```python
from build123d import *

# Parameters (mm, degrees)
F1_DEPTH = 273.05
F2_DEPTH = 6.35
F4_DEPTH = 25.4
F5_W     = 20.32
F5_H     = 203.2
F6_DEPTH = 21.082
F7_R     = 3.175


with BuildPart() as f1:
    # F0 (on Front) → F1 (new body)
    with BuildSketch(Plane.XZ):
        with BuildLine():
            Line((15.875, -3.175), (15.55426, -3.175))
            ThreePointArc((15.55426, -3.175), (10.040232, -12.296722), (0, -15.875))
            Line((0, -15.875), (0, -26.67))
            ThreePointArc((0, -26.67), (8.358623, -25.326317), (15.875, -21.430662))
            Line((15.875, -21.430662), (15.875, -3.175))
        make_face()
        with BuildLine():
            ThreePointArc((0, -15.875), (-10.040232, -12.296722), (-15.55426, -3.175))
            Line((-15.55426, -3.175), (-15.875, -3.175))
            Line((-15.875, -3.175), (-15.875, -21.430662))
            ThreePointArc((-15.875, -21.430662), (-8.358623, -25.326317), (0, -26.67))
            Line((0, -26.67), (0, -15.875))
        make_face()
        with BuildLine():
            ThreePointArc((15.875, -21.430662), (8.358623, -25.326317), (0, -26.67))
            Line((0, -26.67), (0, -27.432))
            ThreePointArc((0, -27.432), (4.143033, -27.930592), (8.049481, -29.397895))
            ThreePointArc((8.049481, -29.397895), (12.080918, -27.983599), (15.875, -26.019508))
            Line((15.875, -26.019508), (15.875, -21.430662))
        make_face()
        with BuildLine():
            ThreePointArc((-8.049481, -29.397895), (-12.080918, -27.983599), (-15.875, -26.019508))
            Line((-15.875, -26.019508), (-15.875, -34.925))
            Line((-15.875, -34.925), (-14.336944, -34.925))
            ThreePointArc((-14.336944, -34.925), (-11.529321, -31.779102), (-8.049481, -29.397895))
        make_face()
        with BuildLine():
            Line((0, -27.432), (0, -26.67))
            ThreePointArc((0, -26.67), (-8.358623, -25.326317), (-15.875, -21.430662))
            Line((-15.875, -21.430662), (-15.875, -26.019508))
            ThreePointArc((-15.875, -26.019508), (-12.080918, -27.983599), (-8.049481, -29.397895))
            ThreePointArc((-8.049481, -29.397895), (-4.143033, -27.930592), (0, -27.432))
        make_face()
        with BuildLine():
            Line((15.875, -34.925), (15.875, -26.019508))
            ThreePointArc((15.875, -26.019508), (12.080918, -27.983599), (8.049481, -29.397895))
            ThreePointArc((8.049481, -29.397895), (11.529321, -31.779102), (14.336944, -34.925))
            Line((14.336944, -34.925), (15.875, -34.925))
        make_face()
        with BuildLine():
            ThreePointArc((0, -12.7), (-7.77713, -10.040232), (-12.296722, -3.175))
            Line((-12.296722, -3.175), (-15.55426, -3.175))
            ThreePointArc((-15.55426, -3.175), (-10.040232, -12.296722), (0, -15.875))
            Line((0, -15.875), (0, -12.7))
        make_face()
        with BuildLine():
            Line((15.55426, -3.175), (12.296722, -3.175))
            ThreePointArc((12.296722, -3.175), (7.77713, -10.040232), (0, -12.7))
            Line((0, -12.7), (0, -15.875))
            ThreePointArc((0, -15.875), (10.040232, -12.296722), (15.55426, -3.175))
        make_face()
    extrude(amount=F1_DEPTH)

    # F0 (on Front) → F2 (join)
    with BuildSketch(Plane.XZ):
        with BuildLine():
            ThreePointArc((0, -12.7), (-7.77713, -10.040232), (-12.296722, -3.175))
            Line((-12.296722, -3.175), (-15.55426, -3.175))
            ThreePointArc((-15.55426, -3.175), (-10.040232, -12.296722), (0, -15.875))
            Line((0, -15.875), (0, -12.7))
        make_face()
        with BuildLine():
            Line((15.55426, -3.175), (12.296722, -3.175))
            ThreePointArc((12.296722, -3.175), (7.77713, -10.040232), (0, -12.7))
            Line((0, -12.7), (0, -15.875))
            ThreePointArc((0, -15.875), (10.040232, -12.296722), (15.55426, -3.175))
        make_face()
    extrude(amount=-F2_DEPTH)

    # F3 (on Right) → F4 (cut, symmetric)
    with BuildSketch(Plane.YZ):
        with BuildLine():
            Line((-285.688049, -3.085141), (-285.688049, -18.728113))
            Line((-285.688049, -18.728113), (-107.888049, -18.728113))
            add(Edge.make_bspline(
                [(-18.988049, -3.085141), (-51.164284, -4.672805), (-75.452253, -18.588752), (-107.888049, -18.728113)],
                knots=[0, 0, 0, 0, 90.265789, 90.265789, 90.265789, 90.265789], degree=3))
            Line((-18.988049, -3.085141), (-285.688049, -3.085141))
        make_face()
    extrude(amount=F4_DEPTH, both=True, mode=Mode.SUBTRACT)

    # F5 (on Top) → F6 (cut)
    with BuildSketch(Plane.XY):
        with Locations((0, -127)):
            Rectangle(F5_W, F5_H)
    extrude(amount=-F6_DEPTH, mode=Mode.SUBTRACT)

    # F7
    f7_edges = [f1.edges().sort_by_distance(p)[0] for p in [
        (-10.16, -25.4, -14.351),
        (10.16, -25.4, -14.351),
        (-10.16, -228.6, -19.905056),
        (10.16, -228.6, -19.905056),
    ]]
    fillet(f7_edges, radius=F7_R)


solid = f1.part
```
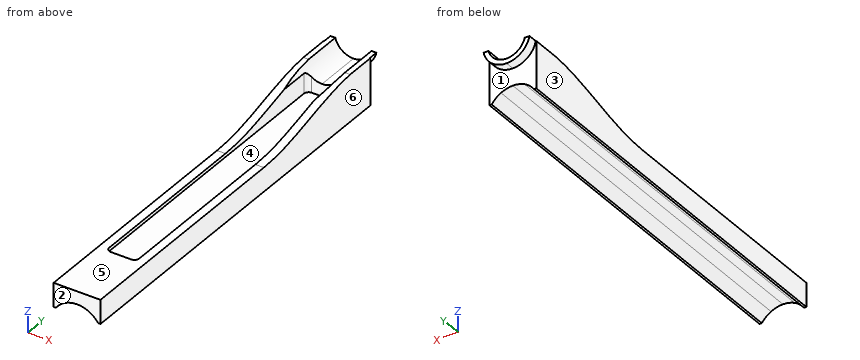
Check sheet for the modelled part. Datum: model origin and axes. Units: mm. Face numbers are marked on the shaded views. A direction names the side the tool comes from. Round coordinates to 2 decimals unless told otherwise and drop trailing zeros. Write each loop counter-clockwise with the first axis right and the second up, starting at its lowest first coordinate (ties: lowest second). Pieces come first, ordered by that corner, then holes. Notation, with made-up numbers: (12.5, 5.5) -> (19.5, 5.5) arc R28 ccw to (19.5, 32.5) -> close; hole circle Ø5 at (-39, 85). An arc over 180 degrees is marked (long way). Put each result on its own line as item: value.
(1) Sectioned sample at A-A (y = -234). Enter the section's corners in (x, z) (1 decimal).
Values found:
outline: (-15.9, -34.9) -> (-14.3, -34.9) arc R17.5 cw to (-8, -29.4) arc R17.5 cw to (0, -27.4) arc R17.5 cw to (8, -29.4) arc R17.5 cw to (14.3, -34.9) -> (15.9, -34.9) -> (15.9, -18.7) -> (-15.9, -18.7) -> close
(2) Mould release check, pull along Y, two halves, no side actions. Record for the marked faces 1, 2, 3 and 4: released by +Y, released by -Y, zero draft, split by the parting line, or undercut.
Values found:
face 1: released by +Y
face 2: released by -Y
face 3: zero draft
face 4: undercut
(3) Sectioned sample at C-C (z = -25). Enter the section's corners in (x, y) (3 decimals), plus the area to 3 significant figures.
Values found:
outline: (-15.875, -273.05) -> (15.875, -273.05) -> (15.875, 0) -> (-15.875, 0) -> close
area: 8,670 mm^2
(4) Tool access check on the marked faces 5 and 6. Record the directions out of +Z, -Z, +X, -X, +Y, -Y that give a thin tool (end or side, any length) a straight path to the whole face; none if there is none.
Values found:
face 5: +Z, +X, -X, -Y
face 6: +Z, -Z, +X, +Y, -Y
(5) Go/stop test with flat-tipped pins: pin 1 Ø4 at (x, y) = (-6, -189) entering from -Z; pin 2 Ø1 at (x, y) = (11, -210) entering from -Z; pin 3 Ø1.9 at (x, z) = (-1, -20) entering from +Y. Record where each tip stops, or that it passes through.
Values found:
pin 1: stops at z = -29.37
pin 2: stops at z = -31.75
pin 3: stops at y = 0
(6) Material ranges on line 1 (X direction, y = -113, z = -32.5) (3 decimals); line 2 (X direction, y = -185.5, z = -19) (3 decimals); line 3 (Y direction, x = -11.5, z = -19), recorded low to high.
Values found:
line 1: x = -15.875 to -12.301, 12.301 to 15.875
line 2: x = -15.875 to -10.16, 10.16 to 15.875
line 3: y = -273.05 to 0
(7) Sectioned sample at B-B (x = 2.5). Enter the section's corners in (y, z).
Values found:
outline: (-273.05, -27.61) -> (0, -27.61) -> (0, -15.68) -> (6.35, -15.68) -> (6.35, -12.45) -> (-25.4, -12.45) -> (-25.4, -21.08) -> (-228.6, -21.08) -> (-228.6, -18.73) -> (-273.05, -18.73) -> close
